Job drawing, mm, ordinate dimensions from the low corner. One solid piece. A direction names the side the tool comes from. Give positions to 0.01 mm unless a question says otherwise; leave off trailing zeros. Write each loop counter-clockwise with the first axis right and the second up, starting at its lowest first coordinate (ties: lowest second). Pieces come first, ordered by that corner, then holes. Notation, with made-up numbers: (45, -37) - (64, -37) arc R16 ccw to (64, -27) - close; hole circle Ø11 at (12.25, 11). An arc over 180 degrees is marked (long way). Put each result on its own line as item: value. Start each with the question number.
1. Drop flat-ended pins along their axis: pin 1 (5.5 mm diameter, centred on x = 44.5, z = 4, fed in from -Y); pin 2 (4 mm diameter, centred on y = 42.5, z = 2.5, fed in from +X); pin 3 (1.5 mm diameter, centred on x = 44, z = 4, fed in from +Y). Give the stop position or say it passes through.
2. Cut at A-A on z = 6.75. List the corners of the cut face in (x, y).
3. Tool access for the marked faces 1, 2 and 3: list every direction of +Z, -Z, +X, -X, +Y, -Y with a clear straight run to the whole face (end or side of a thin tool).
4. Cut at B-B on y = 5.5. List the corners of the cut face in (x, z), and give its area (3 significant figures).
5. Wall check: line 1 (X direction, y = 31.5, z = 6.5); line 2 (Y direction, x = 43.5, z = 5.75). Give the ranges that are in metal, low to high.
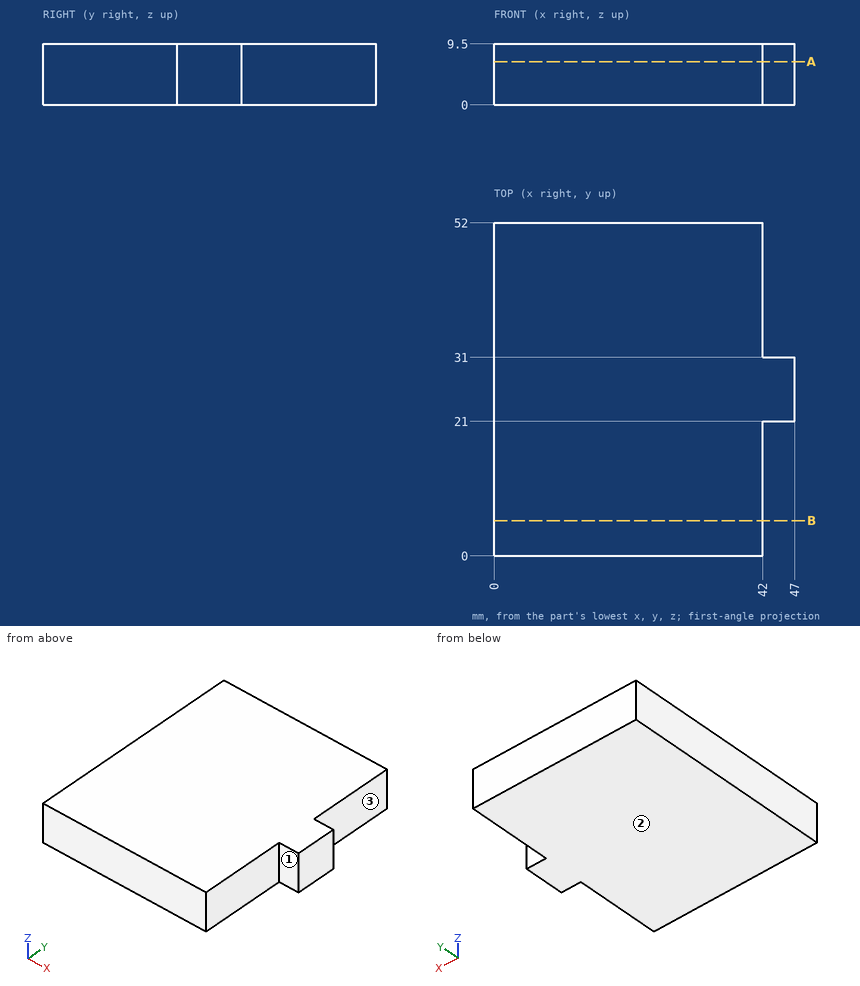
Report:
1. pin 1: stops at y = 0
1. pin 2: stops at x = 42
1. pin 3: stops at y = 31
2. outline: (0, 0) - (42, 0) - (42, 21) - (47, 21) - (47, 31) - (42, 31) - (42, 52) - (0, 52) - close
3. face 1: +Z, -Z, +X, -Y
3. face 2: -Z, +X, -X, +Y, -Y
3. face 3: +Z, -Z, +X, +Y
4. outline: (0, 0) - (42, 0) - (42, 9.5) - (0, 9.5) - close
4. area: 399 mm²
5. line 1: x = 0 to 42
5. line 2: y = 21 to 31
